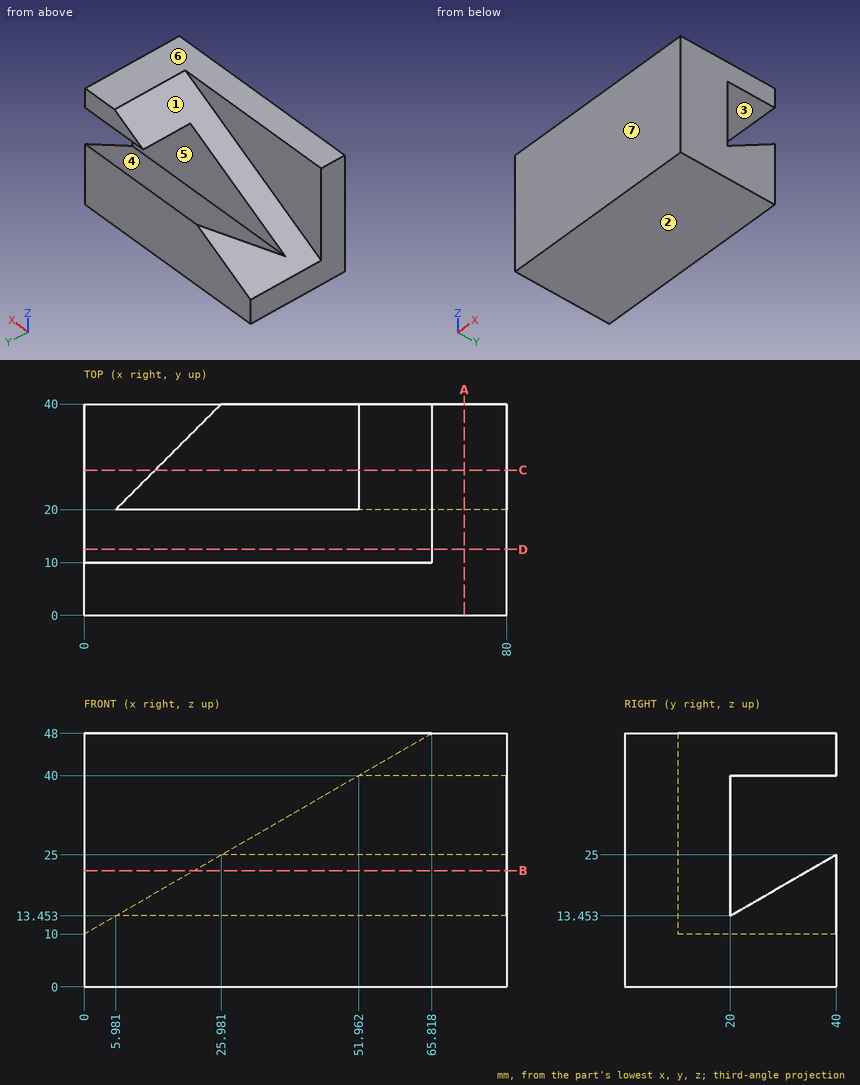
The figure shows three views and two pictorial views of one solid part (mm, origin at its lowest corner). Answer the questions. A direction names the side the tool comes from. Give positions to 0.01 mm unless a question says otherwise; leave off trailing zeros. Write each loop counter-clockwise with the first axis right and the second up, starting at its lowest first coordinate (ties: lowest second). Pieces come first, ordered by that corner, then holes. Notation, with made-up numbers: M 14.5,70.25 L 65.5,70.25 A18 cw 65.5,99.25 Z; hole C 32,-32.75 d5. An arc over 180 degrees is marked long. One line per item, written item: value. Start each with the question number.
(1) Find the intervals of material crossed by line 1 (Y direction, x = 60, z = 21.5) (1 decimal); line 2 (Y direction, x = 68.5, z = 34.5); line 3 (Y direction, x = 20, z = 27), in increasing order.
(2) Find section D-D (y = 12.5). Determine the outline of the cut face in (x, z), plus the area to 3 significant figures.
(3) Find section A-A (x = 72). Determine the outline of the cut face in (y, z).
(4) Flat-ended cylindrical pins translate along their axes: pin 1 Ø2 at (x, y) = (47, 26.5) entering from +Z; pin 2 Ø2 at (y, z) = (31, 16) entering from -X; pin 3 Ø3 at (y, z) = (13, 14) entering from -X. Find the tip coordinate at first contact, or state that the pin passes through.
(5) Find section B-B (z = 22). Determine the outline of the cut face in (x, y) (1 decimal).
(6) A tool of negligible diameter and unlimited length cuts with its end or side. For the marked faces 1, 2 and 3, from which of +Z, -Z, +X, -X, +Y, -Y can it reach the whole face along a straight path? Write none if from no direction.
(7) Find section C-C (y = 27.5). Determine the outline of the cut face in (x, z), plus the area to 3 significant figures.
(8) Determine the mould class of the marked faces 4, 5, 6 and 7 for opening direction Y: pulls with the +Y half, pulls with the -Y half, needs draft (parallel to the pull), parting line crosses it, or undercut.
Results below:
1. line 1: y = 0 to 20, 33.9 to 40
1. line 2: y = 0 to 20
1. line 3: y = 0 to 10
2. outline: M 0,0 L 80,0 L 80,48 L 65.82,48 L 0,10 Z
2. area: 2,590 mm^2
3. outline: M 0,0 L 40,0 L 40,25 L 20,13.45 L 20,40 L 40,40 L 40,48 L 0,48 Z
4. pin 1: stops at z = 17.78
4. pin 2: stops at x = 8.66
4. pin 3: stops at x = 4.33
5. outline: M 0,0 L 80,0 L 80,20 L 20.8,20 L 20.8,10 L 0,10 Z; M 20.8,34.8 L 80,34.8 L 80,40 L 20.8,40 Z
6. face 1: +Z, -X, +Y
6. face 2: -Z, +X, -X, +Y, -Y
6. face 3: +X, -X, +Y
7. outline: M 0,0 L 80,0 L 80,17.78 L 13.48,17.78 L 0,10 Z; M 51.96,40 L 80,40 L 80,48 L 65.82,48 Z
7. area: 1,540 mm^2
8. face 4: undercut
8. face 5: undercut
8. face 6: needs draft
8. face 7: pulls with the -Y half
